```python
from build123d import *

# Parameters (mm, degrees)
SKETCH1_W           = 199
SKETCH1_H           = 45
BOSS_EXTRUDE1_DEPTH = 14
CUT_EXTRUDE1_DEPTH  = 12
CUT_EXTRUDE2_REACH  = 201
SKETCH3_R           = 5.25
SKETCH4_W           = 30
SKETCH4_H           = 15
CUT_EXTRUDE3_DEPTH  = 5
SKETCH5_W           = 199
SKETCH5_H           = 45
SKETCH5_W_2         = 195
SKETCH5_H_2         = 41
BOSS_EXTRUDE2_DEPTH = 10.5
SKETCH6_W           = 1.5
SKETCH6_H           = 2
CUT_EXTRUDE4_DEPTH  = 10.5
BOSS_EXTRUDE5_DEPTH = 41
BOSS_EXTRUDE6_DEPTH = 192
SKETCH9_R           = 3.5
CUT_EXTRUDE5_DEPTH  = 8


with BuildPart() as part:
    # Sketch1 → Boss-Extrude1 (new body)
    with BuildSketch(Plane(origin=(0, 0, 0), x_dir=(1, 0, 0), z_dir=(0, 1, 0))):
        Rectangle(SKETCH1_W, SKETCH1_H)
    extrude(amount=BOSS_EXTRUDE1_DEPTH)

    # Sketch2 → Cut-Extrude1 (cut)
    with BuildSketch(Plane(origin=(0, 14, 0), x_dir=(1, 0, 0), z_dir=(0, 1, 0))):
        Polygon((88.5, 10.5), (88.5, 15.5), (53.5, 15.5), (53.5, -15.5), (88.5, -15.5), (88.5, -10.5), (93.5, -10.5), (93.5, 10.5), align=None)
    extrude(amount=-CUT_EXTRUDE1_DEPTH, mode=Mode.SUBTRACT)

    # Sketch3 → Cut-Extrude2 (cut, up to next)
    with BuildSketch(Plane(origin=(99.5, 0, 0), x_dir=(0, 0, -1), z_dir=(1, 0, 0)), mode=Mode.PRIVATE) as cut_extrude2_sk1:
        with Locations((0, 8)):
            Circle(SKETCH3_R)
    cut_extrude2_tool1 = extrude(cut_extrude2_sk1.sketch, amount=-CUT_EXTRUDE2_REACH, mode=Mode.PRIVATE) & part.part
    add(cut_extrude2_tool1.solids().sort_by_distance((99.5, 8, 0))[0], mode=Mode.SUBTRACT)

    # Sketch4 → Cut-Extrude3 (cut)
    with BuildSketch(Plane(origin=(0, 14, 0), x_dir=(1, 0, 0), z_dir=(0, 1, 0))):
        with Locations((-12.5, 12)):
            Rectangle(SKETCH4_W, SKETCH4_H)
    extrude(amount=-CUT_EXTRUDE3_DEPTH, mode=Mode.SUBTRACT)

    # Sketch5 → Boss-Extrude2 (add)
    with BuildSketch(Plane(origin=(0, 14, 0), x_dir=(1, 0, 0), z_dir=(0, 1, 0))):
        Rectangle(SKETCH5_W, SKETCH5_H)
        Rectangle(SKETCH5_W_2, SKETCH5_H_2, mode=Mode.SUBTRACT)
    extrude(amount=BOSS_EXTRUDE2_DEPTH)

    # Sketch6 → Cut-Extrude4 (cut)
    with BuildSketch(Plane(origin=(0, 24.5, 0), x_dir=(1, 0, 0), z_dir=(0, 1, 0))):
        with Locations((-96.75, 21.5)):
            Rectangle(SKETCH6_W, SKETCH6_H)
        with Locations((96.75, 21.5)):
            Rectangle(SKETCH6_W, SKETCH6_H)
        with Locations((96.75, -21.5)):
            Rectangle(SKETCH6_W, SKETCH6_H)
        with Locations((-96.75, -21.5)):
            Rectangle(SKETCH6_W, SKETCH6_H)
    extrude(amount=-CUT_EXTRUDE4_DEPTH, mode=Mode.SUBTRACT)

    # Sketch7 → Boss-Extrude5 (add)
    with BuildSketch(Plane.XY.offset(-20.5)):
        Polygon((-97.5, 22.500142463), (-96.5, 21.500142463), (-97.5, 20.500142463), align=None)
        Polygon((97.5, 20.500142463), (97.5, 22.500142463), (96.5, 21.500142463), align=None)
    extrude(amount=BOSS_EXTRUDE5_DEPTH)

    # Sketch8 → Boss-Extrude6 (add)
    with BuildSketch(Plane(origin=(96, 0, 0), x_dir=(0, 0, -1), z_dir=(1, 0, 0))):
        Polygon((-20.5, 22.5), (-19.5, 21.5), (-20.5, 20.5), align=None)
        Polygon((20.5, 20.5), (20.5, 22.5), (19.5, 21.5), align=None)
    extrude(amount=-BOSS_EXTRUDE6_DEPTH)

    # Sketch9 → Cut-Extrude5 (cut)
    with BuildSketch(Plane.XZ):
        with Locations((-93.5, 16.5)):
            Circle(SKETCH9_R)
        with Locations((-93.5, -16.5)):
            Circle(SKETCH9_R)
        with Locations((93.5, -16.5)):
            Circle(SKETCH9_R)
        with Locations((93.5, 16.5)):
            Circle(SKETCH9_R)
    extrude(amount=-CUT_EXTRUDE5_DEPTH, mode=Mode.SUBTRACT)


solid = part.part
```
Verification items for the finished model (mm, model axes). A direction names the side the tool comes from. Coordinates: 2 decimals unless noted, no trailing zeros. Order: outer loops, then holes, each group sorted by start corner. A loop starts at its lowest first (then second) coordinate and runs counter-clockwise, first axis right, second up. Notation, with made-up numbers: (5.25, -37) - (58.25, -37) arc R17 ccw to (58.25, -11) - close; hole circle Ø7 at (42.25, 7). An arc over 180 degrees is marked (long way). Return JSON: item names as keys, results as strings.
(1) Access from +Z, -Z, +X, -X, +Y, -Y to the whole of each face (thin tool, end or side, straight path). Record for faces 1 (the flat face through (71, 8, -15.5)), 2 (the cylindrical face through (96.84, 3.94, 17.55)), 3 (the flat face through (-1, 17, 20.5)).
Filled sheet:
{"face 1": "+Y", "face 2": "-Y", "face 3": "none"}
(2) Section check A-A, the plane z = 0. Record the cut outline in (x, y).
Filled sheet:
{"outline": "(-99.5, 0) - (99.5, 0) - (99.5, 2.75) - (93.5, 2.75) - (93.5, 2) - (53.5, 2) - (53.5, 14) - (-97.5, 14) - (-97.5, 20.5) - (-96.5, 21.5) - (-97.5, 22.5) - (-97.5, 24.5) - (-99.5, 24.5) - close; (93.5, 13.25) - (99.5, 13.25) - (99.5, 24.5) - (97.5, 24.5) - (97.5, 22.5) - (96.5, 21.5) - (97.5, 20.5) - (97.5, 14) - (93.5, 14) - close"}
(3) Section check C-C, the plane x = -19.5. Record the cut outline in (y, z), and give its area (3 significant figures).
Filled sheet:
{"outline": "(0, -22.5) - (24.5, -22.5) - (24.5, -20.5) - (22.5, -20.5) - (21.5, -19.5) - (20.5, -20.5) - (14, -20.5) - (14, -19.5) - (9, -19.5) - (9, -4.5) - (14, -4.5) - (14, 20.5) - (20.5, 20.5) - (21.5, 19.5) - (22.5, 20.5) - (24.5, 20.5) - (24.5, 22.5) - (0, 22.5) - close", "area": "599 mm^2"}
(4) Go/stop test with flat-tipped pins: pin 1 (9.5 mm diameter, centred on x = 74, z = -1, fed in from +Y); pin 2 (5.5 mm diameter, centred on x = -93.5, z = 16.5, fed in from -Y); pin 3 (3 mm diameter, centred on x = -73.5, z = -2.5, fed in from +Y). Record where each tip stops, or that it passes through.
Filled sheet:
{"pin 1": "stops at y = 2", "pin 2": "stops at y = 8", "pin 3": "stops at y = 14"}
(5) Mould release check, pull along X, two halves, no side actions. Record for faces 4 (the flat face through (99.5, 15, 0)), 5 (the flat face through (-23, 14, 0)), 6 (the cylindrical face through (96.542, 13.205, 0.683)): pulls with the +X half, pulls with the -X half, needs draft (parallel to the pull), parting line crosses it, or undercut.
Filled sheet:
{"face 4": "pulls with the +X half", "face 5": "undercut", "face 6": "needs draft"}
(6) Thickness scan on line 1 along X through (y, z) = (12.25, -8); line 2 along X through (y, z) = (2.25, -16); line 3 along Z through (x, y) = (-93.5, 2). Record the ranges inside material, lowest first.
Filled sheet:
{"line 1": "x = -99.5 to -27.5, 2.5 to 53.5, 93.5 to 99.5", "line 2": "x = -99.5 to -96.96, -90.04 to 90.04, 96.96 to 99.5", "line 3": "z = -22.5 to -20, -13 to 13, 20 to 22.5"}
(7) Section check B-B, the plane x = -93.5. Record the cut outline in (y, z).
Filled sheet:
{"outline": "(0, -22.5) - (24.5, -22.5) - (24.5, -20.5) - (22.5, -20.5) - (21.5, -19.5) - (20.5, -20.5) - (14, -20.5) - (14, 20.5) - (20.5, 20.5) - (21.5, 19.5) - (22.5, 20.5) - (24.5, 20.5) - (24.5, 22.5) - (0, 22.5) - (0, 20) - (8, 20) - (8, 13) - (0, 13) - (0, -13) - (8, -13) - (8, -20) - (0, -20) - close"}
(8) Section check D-D, the plane x = 69. Record the cut outline in (y, z), and give its area (3 significant figures).
Filled sheet:
{"outline": "(0, -22.5) - (24.5, -22.5) - (24.5, -20.5) - (22.5, -20.5) - (21.5, -19.5) - (20.5, -20.5) - (14, -20.5) - (14, -15.5) - (2, -15.5) - (2, 15.5) - (14, 15.5) - (14, 20.5) - (20.5, 20.5) - (21.5, 19.5) - (22.5, 20.5) - (24.5, 20.5) - (24.5, 22.5) - (0, 22.5) - close", "area": "302 mm^2"}
